from build123d import *

# Parameters (mm, degrees)
SKETCH2_R          = 1.5
CUT_EXTRUDE1_DEPTH = 5
SKETCH3_R          = 1.5
CUT_EXTRUDE2_DEPTH = 25.372115263


with BuildPart() as part:
    # Sketch1 → Revolve1 (revolve)
    with BuildSketch(Plane.XY, mode=Mode.PRIVATE) as revolve1_sk:
        Polygon((12, 3), (12, 15), (8, 15), (8, 5), (1, 5), (0, 4), (0, 3), align=None)
    revolve(revolve1_sk.sketch.rotate(Axis((0, 0, 0), (1, 0, 0)), 90), axis=Axis((0, 0, 0), (1, 0, 0)))

    # Sketch2 → Cut-Extrude1 (cut)
    with BuildSketch(Plane(origin=(0, 0, 0), x_dir=(1, 0, 0), z_dir=(0, 1, 0))):
        with Locations(Location((4, 0, 0), (0, 0, 270))):
            Circle(SKETCH2_R)
    extrude(amount=-CUT_EXTRUDE1_DEPTH, mode=Mode.SUBTRACT)

    # Sketch3 → Cut-Extrude2 (cut, through all)
    with BuildSketch(Plane(origin=(12, 0, 0), x_dir=(0, 0, -1), z_dir=(1, 0, 0))):
        with Locations((-7.071067812, 7.071067812)):
            Circle(SKETCH3_R)
        with Locations((7.071067812, 7.071067812)):
            Circle(SKETCH3_R)
        with Locations((7.071067812, -7.071067812)):
            Circle(SKETCH3_R)
        with Locations((-7.071067812, -7.071067812)):
            Circle(SKETCH3_R)
    extrude(amount=-CUT_EXTRUDE2_DEPTH, mode=Mode.SUBTRACT)


solid = part.part
Verification items for the finished model (mm, model axes). A direction names the side the tool comes from. Give positions to 0.01 mm unless a question says otherwise; leave off trailing zeros. Loops run counter-clockwise (first coordinate to the right, second up) from the corner with the lowest first, then second, coordinate; pieces in that order, holes last.
1) Draft check along X on faces 3 (the cylindrical face through (3.425, -3.783, 1.386)), 4 (the flat face through (8, -4, -4)), 5 (the cylindrical face through (10.028, 7.522, -8.502)). Enter one of: pulls with the +X half, pulls with the -X half, needs draft (parallel to the pull), parting line crosses it, or undercut.
2) Depth check by flat-ended pin: pin 1 Ø4 at (y, z) = (-7.07, -7.07) entering from +X; pin 2 Ø5 at (y, z) = (0, 0) entering from +X; pin 3 Ø2 at (x, z) = (4, 5.5) entering from +Y; pin 4 Ø4 at (y, z) = (7.07, -7.07) entering from -X. Enter the tip coordinate at first touch or a pass-through.
3) Sectioned sample at D-D, the plane z = 6.5. Enter the section's corners in (x, y), then the cut area to 3 significant figures.
4) Sectioned sample at A-A, the plane y = 0. Enter the section's corners in (x, z).
5) Set-up check for faces 1 (the cylindrical face through (10.028, -5.584, 7.266)), 2 (the cylindrical face through (4.45, 4.88, -1.08)): record each of +Z, -Z, +X, -X, +Y, -Y from which the full face is reachable in a straight line by a thin tool's end or side.
6) Thickness scan on line 1 along X through (y, z) = (-10.5, -6); line 2 along Z through (x, y) = (4, -3.25); line 3 along Z through (x, y) = (4, -4.1). Record the ranges inside material, lowest first.
7) Sectioned sample at B-B, the plane z = 0. Enter the section's corners in (x, y).
8) Sectioned sample at C-C, the plane x = 11. Enter the section's corners in (y, z), then the cut area to 3 significant figures.
Answers:
1. face 3: undercut
1. face 4: pulls with the -X half
1. face 5: needs draft
2. pin 1: stops at x = 12
2. pin 2: passes through
2. pin 3: stops at y = 2.18
2. pin 4: stops at x = 8
3. outline: (8, -13.52) - (12, -13.52) - (12, -8.46) - (8, -8.46) - close; (8, -5.68) - (12, -5.68) - (12, 5.68) - (8, 5.68) - close; (8, 8.46) - (12, 8.46) - (12, 13.52) - (8, 13.52) - close
3. area: 86.0 mm2
4. outline: (0, -4) - (1, -5) - (8, -5) - (8, -15) - (12, -15) - (12, -3) - (0, -3) - close; (0, 3) - (12, 3) - (12, 15) - (8, 15) - (8, 5) - (1, 5) - (0, 4) - close
5. face 1: +X, -X
5. face 2: -X
6. line 1: x = 8 to 12
6. line 2: z = -3.8 to -1.5, 1.5 to 3.8
6. line 3: z = -2.86 to -1.5, 1.5 to 2.86
7. outline: (0, -4) - (1, -5) - (2.5, -5) - (2.5, -3) - (0, -3) - close; (0, 3) - (12, 3) - (12, 15) - (8, 15) - (8, 5) - (1, 5) - (0, 4) - close; (5.5, -5) - (8, -5) - (8, -15) - (12, -15) - (12, -3) - (5.5, -3) - close
8. outline: circle Ø30 at (0, 0); hole circle Ø3 at (-7.07, -7.07); hole circle Ø3 at (-7.07, 7.07); hole circle Ø6 at (0, 0); hole circle Ø3 at (7.07, -7.07); hole circle Ø3 at (7.07, 7.07)
8. area: 650 mm2
